```python
from build123d import *

# Parameters (mm, degrees)
MODEL_W                 = 10
MODEL_H                 = 3
MODEL_W_2               = 3
MODEL_H_2               = 5
SALIENTE_EXTRUIR1_DEPTH = 3


with BuildPart() as part:
    # Model → Saliente-Extruir1 (new body)
    with BuildSketch(Plane.XY):
        with BuildLine():
            Line((91.780211275, 65.839195147), (91.780211275, 57.379955116))
            Line((91.780211275, 57.379955116), (91.780211275, 13.141428354))
            Line((91.780211275, 13.141428354), (91.780211275, 3.638851328))
            Line((91.780211275, 3.638851328), (91.780211275, -1.666158522))
            ThreePointArc((91.780211275, -1.666158522), (90.315745044, -5.201692177), (86.780211275, -6.666158134))
            Line((86.780211275, -6.666158134), (14.78327762, -6.666158134))
            ThreePointArc((14.78327762, -6.666158134), (11.247743714, -5.20169204), (9.78327762, -1.666158134))
            Line((9.78327762, -1.666158134), (9.78327762, 23.733841478))
            Line((9.78327762, 23.733841478), (9.78327762, 46.933841478))
            Line((9.78327762, 46.933841478), (9.78327762, 77.517630631))
            Line((9.78327762, 77.517630631), (9.78327762, 85.517630631))
            ThreePointArc((9.78327762, 85.517630631), (11.247743714, 89.053164537), (14.78327762, 90.517630631))
            Line((14.78327762, 90.517630631), (86.780211275, 90.517630631))
            ThreePointArc((86.780211275, 90.517630631), (90.315745181, 89.053164537), (91.780211275, 85.517630631))
            Line((91.780211275, 85.517630631), (91.77714493, 80.517630631))
            Line((91.77714493, 80.517630631), (91.780211275, 65.839195147))
        make_face()
        with Locations((64.780211275, 84.017630631)):
            Rectangle(MODEL_W, MODEL_H, mode=Mode.SUBTRACT)
        with Locations((36.780211275, 84.017630631)):
            Rectangle(MODEL_W, MODEL_H, mode=Mode.SUBTRACT)
        with Locations((75.880211275, 42.833841478)):
            Rectangle(MODEL_W_2, MODEL_H_2, mode=Mode.SUBTRACT)
        with Locations((75.880211275, 27.833841478)):
            Rectangle(MODEL_W_2, MODEL_H_2, mode=Mode.SUBTRACT)
        with Locations((15.68327762, 42.833841478)):
            Rectangle(MODEL_W_2, MODEL_H_2, mode=Mode.SUBTRACT)
        with Locations((15.68327762, 27.833841478)):
            Rectangle(MODEL_W_2, MODEL_H_2, mode=Mode.SUBTRACT)
        with Locations((85.880211275, 42.833841478)):
            Rectangle(MODEL_W_2, MODEL_H_2, mode=Mode.SUBTRACT)
        with Locations((85.880211275, 27.833841478)):
            Rectangle(MODEL_W_2, MODEL_H_2, mode=Mode.SUBTRACT)
        with Locations((25.68327762, 42.833841478)):
            Rectangle(MODEL_W_2, MODEL_H_2, mode=Mode.SUBTRACT)
        with Locations((25.68327762, 27.833841478)):
            Rectangle(MODEL_W_2, MODEL_H_2, mode=Mode.SUBTRACT)
    extrude(amount=SALIENTE_EXTRUIR1_DEPTH)


solid = part.part
```
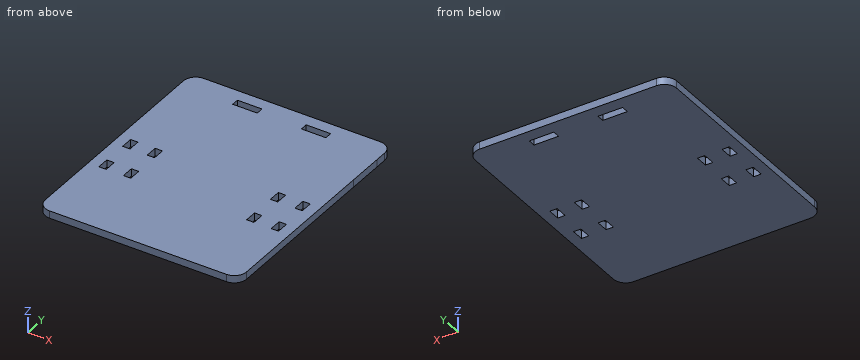
Check sheet for the modelled part. Datum: model origin and axes. Units: mm. Round coordinates to 2 decimals unless told otherwise and drop trailing zeros. Loops run counter-clockwise (first coordinate to the right, second up) from the corner with the lowest first, then second, coordinate; pieces in that order, holes last. Notation, with made-up numbers: (14.25, 31.5) - (71.25, 31.5) arc R33 cw to (71.25, 60.5) - close; hole circle Ø3 at (-23, 87.25). An arc over 180 degrees is marked (long way). Answer as a JSON object with one key per item and string values. Group by question number.
Q1. Sectioned sample at A-A, the plane x = 65.5. Enter the section's corners in (y, z).
Q2. Scan lines: line 1 along Y through (x, z) = (86.5, 1.9); line 2 along Y through (x, z) = (41, 0.15). Record each from-to range of solid material in increasing order. Write a range as [from, to].
Q3. Sectioned sample at B-B, the plane z = 2.2. Count the separate pieces of the cut face and the enclosed holes in it, plus the area to 3 significant figures.
Solution:
{
 "1": {"outline": "(-6.67, 0) - (82.52, 0) - (82.52, 3) - (-6.67, 3) - close; (85.52, 0) - (90.52, 0) - (90.52, 3) - (85.52, 3) - close"},
 "2": {"line 1": "y = [-6.67, 25.33], [30.33, 40.33], [45.33, 90.52]", "line 2": "y = [-6.67, 82.52], [85.52, 90.52]"},
 "3": {"separate pieces": "1", "enclosed holes": "10", "area": "7,770 mm²"}
}
